Check sheet for the modelled part. Datum: model origin and axes. Units: mm. Round coordinates to 2 decimals unless told otherwise and drop trailing zeros. Write each loop counter-clockwise with the first axis right and the second up, starting at its lowest first coordinate (ties: lowest second). Pieces come first, ordered by that corner, then holes. Notation, with made-up numbers: (-16, 48.5) - (-4, 48.5) arc R18 cw to (-4, 60.5) - close; hole circle Ø5 at (-16.75, 62.25). An arc over 180 degrees is marked (long way). Use one line per item in the form item = value. Start each with the question number.
1) Section check A-A (y = 4.5). Count the separate pieces of the cut face and the enclosed holes in it, then the cut area to 3 significant figures.
2) Section check B-B (x = 113). Record the boundary of the cut face in (y, z), then the cut area to 3 significant figures.
3) Gauge pin test, flat ends, axial feed: P1, Ø3, axis at y = 2, z = -630, coming from the -X side; P2, Ø1.5, axis at y = 5.5, z = -372.5, coming from the +X side; P3, Ø2, axis at x = 158.5, y = 2, coming from the +Z side. Record the tip position at first contact, or that the pin passes through.
4) Section check C-C (z = -281.5). Record the boundary of the cut face in (x, y), then the cut area to 3 significant figures.
5) Scan lines: probe 1 along X at (y, z) = (0.75, -627.5) (3 decimals); probe 2 along X at (y, z) = (3, -8); probe 3 along X at (y, z) = (3.5, -307.5). Record each from-to range of solid material in increasing order.
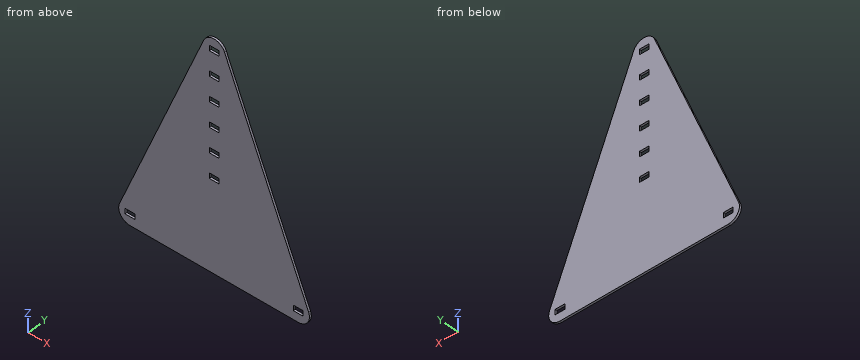
from build123d import *

# Parameters (mm, degrees)
SKETCH1_W           = 30
SKETCH1_H           = 16.5
BOSS_EXTRUDE1_DEPTH = 6.35


with BuildPart() as part:
    # Sketch1 → Boss-Extrude1 (new body)
    with BuildSketch(Plane(origin=(0, 0, 0), x_dir=(1, 0, 0), z_dir=(0, 1, 0))):
        with BuildLine():
            Line((32.354745971, -13.34804904), (293.859745971, 620.52195096))
            ThreePointArc((293.859745971, 620.52195096), (290.592640987, 653.335588658), (261.505, 668.87))
            Line((261.505, 668.87), (-261.505, 668.87))
            ThreePointArc((-261.505, 668.87), (-290.592640987, 653.335588658), (-293.859745971, 620.52195096))
            Line((-293.859745971, 620.52195096), (-32.354745971, -13.34804904))
            ThreePointArc((-32.354745971, -13.34804904), (0, -35), (32.354745971, -13.34804904))
        make_face()
        with Locations((0, 76.5)):
            Rectangle(SKETCH1_W, SKETCH1_H, mode=Mode.SUBTRACT)
        with Locations((261.505, 633.87)):
            Rectangle(SKETCH1_W, SKETCH1_H, mode=Mode.SUBTRACT)
        Rectangle(SKETCH1_W, SKETCH1_H, mode=Mode.SUBTRACT)
        with Locations((0, 153)):
            Rectangle(SKETCH1_W, SKETCH1_H, mode=Mode.SUBTRACT)
        with Locations((0, 229.5)):
            Rectangle(SKETCH1_W, SKETCH1_H, mode=Mode.SUBTRACT)
        with Locations((0, 306)):
            Rectangle(SKETCH1_W, SKETCH1_H, mode=Mode.SUBTRACT)
        with Locations((0, 382.5)):
            Rectangle(SKETCH1_W, SKETCH1_H, mode=Mode.SUBTRACT)
        with Locations((-261.505, 633.87)):
            Rectangle(SKETCH1_W, SKETCH1_H, mode=Mode.SUBTRACT)
    extrude(amount=BOSS_EXTRUDE1_DEPTH)


solid = part.part
Results are:
q1.separate_pieces = 1
q1.enclosed_holes = 8
q1.area = 232,000 mm²
q2.outline = (0, -668.87) - (6.35, -668.87) - (6.35, -182.13) - (0, -182.13) - close
q2.area = 3,090 mm²
q3.P1 = -296.42
q3.P2 = 191.85
q3.P3 = -290
q4.outline = (-154, 0) - (154, 0) - (154, 6.35) - (-154, 6.35) - close
q4.area = 1,960 mm²
q5.probe_1 = -295.92 to -276.505, -246.505 to 246.505, 276.505 to 295.92
q5.probe_2 = -41.16 to -15, 15 to 41.16
q5.probe_3 = -164.72 to -15, 15 to 164.72
